```python
from build123d import *

# Parameters (mm, degrees)
F0_R      = 30
F3_R      = 30
F0_R_2    = 82.5
F5_DEPTH  = 15
F6_R      = 9
F7_DEPTH  = 25
F8_R      = 82.5
F8_R_2    = 9
F8_R_3    = 30
F9_DEPTH  = 15
F10_R     = 82.5
F10_R_2   = 9
F10_R_3   = 30
F11_DEPTH = 15
F12_R     = 25
F13_DEPTH = 368.6303645372


with BuildPart() as f2:
    # F2: sweep along a path in F1
    with BuildLine(Plane.YZ) as f2_path:
        Line((0, 0), (-255, 0))
        ThreePointArc((-255, 0), (-325.7106781187, -29.2893218813), (-355, -100))
        Line((-355, -100), (-355, -693))
        Line((-355, -693), (-547.1918582916, -693))
    # F0 (on Front) → F2 (sweep)
    with BuildSketch(Plane.XZ):
        Circle(F0_R)
    sweep(path=f2_path.line, transition=Transition.RIGHT)

    # F4: sweep along a path in F1
    with BuildLine(Plane.YZ) as f4_path:
        Line((-547.1918582916, -693), (-355, -693))
        Line((-355, -693), (-178.5614937544, -693))
    # F3 (on face) → F4 (sweep)
    with BuildSketch(Plane.XZ.offset(547.1918582916)):
        with Locations((0, -693)):
            Circle(F3_R)
    sweep(path=f4_path.line)

    # F0 (on Front) → F5 (join)
    with BuildSketch(Plane.XZ):
        Circle(F0_R_2)
        Circle(F0_R, mode=Mode.SUBTRACT)
    extrude(amount=F5_DEPTH)

    # F6 (on face) → F7 (cut)
    with BuildSketch(Plane.XZ):
        with Locations((0, 62.5)):
            Circle(F6_R)
        with Locations((-62.5, 0)):
            Circle(F6_R)
        with Locations((0, -62.5)):
            Circle(F6_R)
        with Locations((62.5, 0)):
            Circle(F6_R)
    extrude(amount=F7_DEPTH, mode=Mode.SUBTRACT)

    # F8 (on face) → F9 (join)
    with BuildSketch(Plane.XZ.offset(547.1918582916)):
        with Locations((0, -693)):
            Circle(F8_R)
        with Locations((0, -755.5)):
            Circle(F8_R_2, mode=Mode.SUBTRACT)
        with Locations((-62.5, -693)):
            Circle(F8_R_2, mode=Mode.SUBTRACT)
        with Locations((0, -693)):
            Circle(F8_R_3, mode=Mode.SUBTRACT)
        with Locations((62.5, -693)):
            Circle(F8_R_2, mode=Mode.SUBTRACT)
        with Locations((0, -630.5)):
            Circle(F8_R_2, mode=Mode.SUBTRACT)
    extrude(amount=-F9_DEPTH)

    # F10 (on face) → F11 (join)
    with BuildSketch(Plane(origin=(0, -178.5614937544, 0), x_dir=(-1, 0, 0), z_dir=(0, 1, 0))):
        with Locations((0, -693)):
            Circle(F10_R)
        with Locations((0, -755.5)):
            Circle(F10_R_2, mode=Mode.SUBTRACT)
        with Locations((-62.5, -693)):
            Circle(F10_R_2, mode=Mode.SUBTRACT)
        with Locations((0, -693)):
            Circle(F10_R_3, mode=Mode.SUBTRACT)
        with Locations((62.5, -693)):
            Circle(F10_R_2, mode=Mode.SUBTRACT)
        with Locations((0, -630.5)):
            Circle(F10_R_2, mode=Mode.SUBTRACT)
    extrude(amount=-F11_DEPTH)

    # F12 (on face) → F13 (cut, through all)
    with BuildSketch(Plane(origin=(0, -178.5614937544, 0), x_dir=(-1, 0, 0), z_dir=(0, 1, 0))):
        with Locations((0, -693)):
            Circle(F12_R)
    extrude(amount=-F13_DEPTH, mode=Mode.SUBTRACT)


solid = f2.part
```
Could you check a few things on this model? Use its own coordinates, in mm. A direction names the side the tool comes from. Round coordinates to 2 decimals unless told otherwise and drop trailing zeros. Write each loop counter-clockwise with the first axis right and the second up, starting at its lowest first coordinate (ties: lowest second). Pieces come first, ordered by that corner, then holes. Notation, with made-up numbers: M -2,-23.5 L 3,-23.5 A12 cw 3,-14.5 Z; hole C 12,87.5 d10. An arc over 180 degrees is marked long. Write each question's results on one line, items separated by ' | '. Start each with the question number.
1. I need wall thicknesses on L1, parallel to Z at x = 0, y = -3; L2, parallel to Z at x = 0, y = -537; L3, parallel to Y at x = 62, z = -676. Which ranges of each line are inside material? Lowest first, please. Write a range as from..to.
2. Imagine slicing it at C-C on x = 62.5. List the corners of the cut face in (y, z) for me, and give its area (3 significant figures).
3. Thinking about a two-plate mould opening in X: for faces 4 (the face through (-17.88, -7.4, -80.54)), 5 (the face through (36, -532.192, -692)), 6 (the face through (71.084, -7.395, 2.703)), which applies, +X half, -X half, draft (parallel to the pull), parting line (faces both ways), or undercut?
4. I'm going to push flat-ended pins straight in: pin 1 Ø23.5 at (x, z) = (0, -630.5) entering from +Y; pin 2 Ø11 at (x, z) = (0, -630.5) entering from -Y; pin 3 Ø11 at (x, z) = (62.5, -693) entering from +Y; pin 4 Ø1 at (x, z) = (20.5, -143) entering from -Y. Where does each tip first touch, or does it pass through?
5. On a 3-axis mill with a long thin cutter (end or side, diameter ignored), from which of +Z, -Z, +X, -X, +Y, -Y can I reach the whole of each face in a straight line? I mean faces 1 (the face through (-1.951, -7.395, -71.286)), 2 (the face through (-29.97, -136.68, 1.32)), 3 (the face through (19, -178.561, -710)). Say none if no direction works.
6. Imagine slicing it at A-A on y = -202. List the corners of the cut face in (x, z) for me.
7. Imagine slicing it at B-B on z = 62.5. List the corners of the cut face in (x, y) for me, and give its area (3 significant figures).
8. Imagine slicing it at D-D on z = -755.5. List the corners of the cut face in (x, y) for me, and give its area (3 significant figures).
Result sheet:
1) L1: z = -82.5..-71.5, -53.5..53.5, 71.5..82.5 | L2: z = -775.5..-764.5, -746.5..-718, -668..-639.5, -621.5..-610.5 | L3: y = -547.19..-532.19, -193.56..-178.56
2) outline: M -547.19,-746.85 L -532.19,-746.85 L -532.19,-702 L -547.19,-702 Z; M -547.19,-684 L -532.19,-684 L -532.19,-639.15 L -547.19,-639.15 Z; M -193.56,-746.85 L -178.56,-746.85 L -178.56,-702 L -193.56,-702 Z; M -193.56,-684 L -178.56,-684 L -178.56,-639.15 L -193.56,-639.15 Z; M -15,-53.85 L 0,-53.85 L 0,-9 L -15,-9 Z; M -15,9 L 0,9 L 0,53.85 L -15,53.85 Z | area: 4,040 mm^2
3) face 4: parting line | face 5: draft | face 6: undercut
4) pin 1: stops at y = -178.56 | pin 2: stops at y = -385 | pin 3: passes through | pin 4: stops at y = -377.36
5) face 1: +Y | face 2: none | face 3: -Z, +X, -X, +Y
6) outline: C 0,-693 d60; C 0,0 d60; hole C 0,-693 d50
7) outline: M -53.85,-15 L -9,-15 L -9,0 L -53.85,0 Z; M 9,-15 L 53.85,-15 L 53.85,0 L 9,0 Z | area: 1,350 mm^2
8) outline: M -53.85,-547.19 L -9,-547.19 L -9,-532.19 L -53.85,-532.19 Z; M -53.85,-193.56 L -9,-193.56 L -9,-178.56 L -53.85,-178.56 Z; M 9,-547.19 L 53.85,-547.19 L 53.85,-532.19 L 9,-532.19 Z; M 9,-193.56 L 53.85,-193.56 L 53.85,-178.56 L 9,-178.56 Z | area: 2,690 mm^2
